```python
from build123d import *

# Parameters (mm, degrees)
SKETCH1_R           = 13.5
BOSS_EXTRUDE1_DEPTH = 7
SKETCH2_R           = 16.5
BOSS_EXTRUDE2_DEPTH = 1.5
BOSS_EXTRUDE3_START = 1.5
SKETCH3_R           = 16.5
BOSS_EXTRUDE3_DEPTH = 1.5
SKETCH4_R           = 6.5
CUT_EXTRUDE1_DEPTH  = 26.38700455
SKETCH5_R           = 6.5
SKETCH5_R_2         = 2.25
BOSS_EXTRUDE4_DEPTH = 2.5


with BuildPart() as part:
    # Sketch1 → Boss-Extrude1 (new body)
    with BuildSketch(Plane.XY):
        Circle(SKETCH1_R)
    extrude(amount=BOSS_EXTRUDE1_DEPTH)

    # Sketch2 → Boss-Extrude2 (add)
    with BuildSketch(Plane.XY.offset(7)):
        Circle(SKETCH2_R)
    extrude(amount=BOSS_EXTRUDE2_DEPTH)

    # Sketch3 → Boss-Extrude3 (add)
    with BuildSketch(Plane(origin=(0, 0, 0), x_dir=(-1, 0, 0), z_dir=(0, 0, -1)).offset(BOSS_EXTRUDE3_START)):
        with Locations(Location((0, 0, 0), (0, 0, 180))):
            Circle(SKETCH3_R)
    extrude(amount=-BOSS_EXTRUDE3_DEPTH)

    # Sketch4 → Cut-Extrude1 (cut, through all)
    with BuildSketch(Plane.XY.offset(8.5)):
        Circle(SKETCH4_R)
    extrude(amount=-CUT_EXTRUDE1_DEPTH, mode=Mode.SUBTRACT)

    # Sketch5 → Boss-Extrude4 (add)
    with BuildSketch(Plane.XY.offset(8.5)):
        Circle(SKETCH5_R)
        Circle(SKETCH5_R_2, mode=Mode.SUBTRACT)
    extrude(amount=-BOSS_EXTRUDE4_DEPTH)


solid = part.part
```
The listing builds one solid part. Answer for the finished solid, in the listing's coordinates (mm). A direction names the side the tool comes from. Give positions to 0.01 mm unless a question says otherwise; leave off trailing zeros. Write each loop counter-clockwise with the first axis right and the second up, starting at its lowest first coordinate (ties: lowest second). Pieces come first, ordered by that corner, then holes. Notation, with made-up numbers: (-36, 78) -> (-19, 78) arc R23 ccw to (-19, 92) -> close; hole circle Ø5 at (68.5, 20). An arc over 180 degrees is marked (long way). Use one line per item in the form item = value.
1) Section C-C on z = 4.5 is taken. Write down the section's boundary in (x, y).
Result:
outline = circle Ø27 at (0, 0); hole circle Ø13 at (0, 0)
2) A tool of negligible diameter and unlimited length cuts with its end or side. For faces 4 (the cylindrical face through (-5.158, -3.955, 2.302)), 5 (the flat face through (0, 7, -1.5)), 6 (the flat face through (-14, 0, 0)), from which of +Z, -Z, +X, -X, +Y, -Y can it reach the whole face along a straight path? Write none if from no direction.
Result:
face_4 = -Z
face_5 = -Z, +X, -X, +Y, -Y
face_6 = none
3) For a pull along X with two mould halves and no side action, classify faces 1 (the flat face through (3, 0, 6)), 2 (the flat face through (-14, 0, 7)), 3 (the cylindrical face through (-2.93, -13.18, 3.45)) as +X half, -X half, draft (parallel to the pull), parting line (faces both ways), or undercut.
Result:
face_1 = undercut
face_2 = draft
face_3 = parting line
4) Each of these flat-tipped pins is pushed along its axis until it touches: P1, Ø8, axis at x = 2.5, y = 1.5, coming from the -Z side; P2, Ø1.5, axis at x = 7.5, z = 7, coming from the -Y side; P3, Ø4, axis at y = 6.5, z = 6.5, coming from the +X side; P4, Ø1.5, axis at x = 11.5, z = 0.5, coming from the +Y side. Where does it stop, or does it pass through?
Result:
P1 = -1.5
P2 = -15.06
P3 = 15.86
P4 = 12.35
5) Straight lines are drawn through the part: probe 1 along Y at (x, z) = (0, 7.2); probe 2 along Y at (x, z) = (0, 4.25); probe 3 along Z at (x, y) = (-3, 3.5). For each, find the intervals that lie inside material, in ascending order.
Result:
probe_1 = -16.5 to -2.25, 2.25 to 16.5
probe_2 = -13.5 to -6.5, 6.5 to 13.5
probe_3 = 6 to 8.5
6) Section A-A on x = 0 is taken. Write down the section's boundary in (y, z).
Result:
outline = (-16.5, -1.5) -> (-6.5, -1.5) -> (-6.5, 6) -> (-2.25, 6) -> (-2.25, 8.5) -> (-16.5, 8.5) -> (-16.5, 7) -> (-13.5, 7) -> (-13.5, 0) -> (-16.5, 0) -> close; (2.25, 6) -> (6.5, 6) -> (6.5, -1.5) -> (16.5, -1.5) -> (16.5, 0) -> (13.5, 0) -> (13.5, 7) -> (16.5, 7) -> (16.5, 8.5) -> (2.25, 8.5) -> close
7) Section D-D on x = -11.5 is taken. Write down the section's boundary in (y, z).
Result:
outline = (-11.83, -1.5) -> (11.83, -1.5) -> (11.83, 0) -> (7.07, 0) -> (7.07, 7) -> (11.83, 7) -> (11.83, 8.5) -> (-11.83, 8.5) -> (-11.83, 7) -> (-7.07, 7) -> (-7.07, 0) -> (-11.83, 0) -> close
